Model file for the job. Use its own axes, mm. A direction names the side the tool comes from. Round coordinates to 2 decimals unless told otherwise and drop trailing zeros. Order: outer loops, then holes, each group sorted by start corner. A loop starts at its lowest first (then second) coordinate and runs counter-clockwise, first axis right, second up. Notation, with made-up numbers: (25.25, -4) - (73.25, -4) arc R10 cw to (73.25, 0) - close; hole circle Ø5 at (11.5, -38.5). An arc over 180 degrees is marked (long way). Answer as CSV lines item,"result". Start each with the question number.
1. Band-saw the part on C-C on y = -62. List the corners of the cut face in (x, z), then the cut area to 3 significant figures.
2. Pin check, flat tips, straight feed: pin 1 Ø1.5 at (x, z) = (2, 44) entering from +Y; pin 2 Ø3 at (y, z) = (-21.5, 20.5) entering from -X; pin 3 Ø1.5 at (x, y) = (1.5, -30) entering from +Z; pin 4 Ø1.5 at (x, z) = (3, -15.5) entering from +Y (3 decimals). Stop position of each tip, or through.
3. Band-saw the part on A-A on z = 45.5. List the corners of the cut face in (x, y), then the cut area to 3 significant figures.
4. Band-saw the part on D-D on y = -33. List the corners of the cut face in (x, z), then the cut area to 3 significant figures.
5. Wall check: line 1 along Y through (x, z) = (4, 0); line 2 along Z through (x, y) = (1, -30); line 3 along Y through (x, z) = (2.7, -17). Give the ranges that are in metal, low to high. Write a range as [from, to].
6. Band-saw the part on B-B on y = -17. List the corners of the cut face in (x, z), then the cut area to 3 significant figures.
7. 3-axis set-ups, long thin cutter, end or side, ignore diameter. For faces 1 (the face through (3, -34, 25.706)), 2 (the face through (5, -28.6, 7.8)): which of +Z, -Z, +X, -X, +Y, -Y reach the whole face in a straight line?
8. Pull direction Z, two halves, no side cores. Call faces 3 (the face through (2.54, -56.43, -11.4)), 4 (the face through (2, -32, -27)), 5 (the face through (3, -65, 19)): released by +Z, released by -Z, zero draft, split by the parting line, or undercut.
```python
from build123d import *

# Parameters (mm, degrees)
SKETCH_1_R           = 27
SKETCH_1_R_2         = 18.5
EXTRUDE_1_DEPTH      = 5
SKETCH_2_R           = 1.6
CUT_EXTRUDE_1_DEPTH  = 10
EXTRUDE_2_DEPTH      = 5
SKETCH_9_W           = 91
SKETCH_9_H           = 135
CUT_EXTRUDE_5_DEPTH  = 211.049994049
SKETCH_13_R          = 2.1
SKETCH_13_R_2        = 3.0525
CUT_EXTRUDE_6_DEPTH  = 92.356444764
SKETCH_14_R          = 1.6
CUT_EXTRUDE_7_DEPTH  = 92.356444764
SKETCH_15_W          = 24
SKETCH_15_H          = 9
CUT_EXTRUDE_8_DEPTH  = 10
FILLET_1_R           = 2
CUT_EXTRUDE_9_DEPTH  = 92.356444764
FILLET_2_R           = 1.3
CUT_EXTRUDE_10_DEPTH = 92.356444764
FILLET_3_R           = 1.3


with BuildPart() as part:
    # 草图1 → 凸台-拉伸1 (new body)
    with BuildSketch(Plane(origin=(0, 0, 0), x_dir=(0, 0, -1), z_dir=(1, 0, 0))):
        Circle(SKETCH_1_R)
        Circle(SKETCH_1_R_2, mode=Mode.SUBTRACT)
    extrude(amount=EXTRUDE_1_DEPTH)

    # 草图2 → 切除-拉伸1 (cut)
    with BuildSketch(Plane(origin=(5, 0, 0), x_dir=(0, 0, -1), z_dir=(1, 0, 0))):
        with Locations((23, 0)):
            Circle(SKETCH_2_R)
        with Locations((0, -23)):
            Circle(SKETCH_2_R)
        with Locations((0, 23)):
            Circle(SKETCH_2_R)
        with Locations((-23, 0)):
            Circle(SKETCH_2_R)
    extrude(amount=-CUT_EXTRUDE_1_DEPTH, mode=Mode.SUBTRACT)

    # 草图3 → 凸台-拉伸2 (add)
    with BuildSketch(Plane.ZY):
        with BuildLine():
            ThreePointArc((27, 0), (0, -27), (-27, 0))
            Line((-27, 0), (-27, -200))
            Line((-27, -200), (64, -200))
            Line((64, -200), (64, -60))
            Line((64, -60), (23.632414536, 13.057908838))
            ThreePointArc((23.632414536, 13.057908838), (26.144551942, 6.742581388), (27, 0))
        make_face()
    extrude(amount=-EXTRUDE_2_DEPTH)

    # 草图9 → 切除-拉伸5 (cut, through all)
    with BuildSketch(Plane(origin=(5, 0, 0), x_dir=(0, 0, -1), z_dir=(1, 0, 0))):
        with Locations((-18.5, -132.5)):
            Rectangle(SKETCH_9_W, SKETCH_9_H)
    extrude(amount=-CUT_EXTRUDE_5_DEPTH, mode=Mode.SUBTRACT)

    # 草图13 → 切除-拉伸6 (cut, through all)
    with BuildSketch(Plane(origin=(5, 0, 0), x_dir=(0, 0, -1), z_dir=(1, 0, 0))):
        with Locations((-17.5, -45)):
            Circle(SKETCH_13_R)
        with Locations((-17.5, -60)):
            Circle(SKETCH_13_R_2)
        with Locations((17.5, -60)):
            Circle(SKETCH_13_R_2)
        with Locations((17.5, -45)):
            Circle(SKETCH_13_R)
    extrude(amount=-CUT_EXTRUDE_6_DEPTH, mode=Mode.SUBTRACT)

    # 草图14 → 切除-拉伸7 (cut, through all)
    with BuildSketch(Plane.ZY):
        with Locations((39, -62)):
            Circle(SKETCH_14_R)
        with Locations((59, -62)):
            Circle(SKETCH_14_R)
    extrude(amount=-CUT_EXTRUDE_7_DEPTH, mode=Mode.SUBTRACT)

    # 草图15 → 切除-拉伸8 (cut)
    with BuildSketch(Plane.ZY):
        with Locations((0, -52.5)):
            Rectangle(SKETCH_15_W, SKETCH_15_H)
    extrude(amount=-CUT_EXTRUDE_8_DEPTH, mode=Mode.SUBTRACT)

    # 圆角1
    fillet_1_edges = [part.edges().sort_by_distance(p)[0] for p in [
        (2.5, -57, -12),
        (2.5, -48, -12),
        (2.5, -48, 12),
        (2.5, -57, 12),
    ]]
    fillet(fillet_1_edges, radius=FILLET_1_R)

    # 草图16 → 切除-拉伸9 (cut, through all)
    with BuildSketch(Plane(origin=(5, 0, 0), x_dir=(0, 0, -1), z_dir=(1, 0, 0))):
        with BuildLine():
            Line((-28.536090226, -9.256973298), (-52.705963097, -53))
            Line((-52.705963097, -53), (-25.705963097, -53))
            Line((-25.705963097, -53), (-25.705963097, -15.466203841))
            ThreePointArc((-25.705963097, -15.466203841), (-27.29814505, -12.442317985), (-28.536090226, -9.256973298))
        make_face()
    extrude(amount=-CUT_EXTRUDE_9_DEPTH, mode=Mode.SUBTRACT)

    # 圆角2
    fillet_2_edges = [part.edges().sort_by_distance(p)[0] for p in [
        (2.5, -9.256973298, 28.536090226),
        (2.5, -15.466203841, 25.705963097),
        (2.5, -53, 25.705963097),
        (2.5, -53, 52.705963097),
    ]]
    fillet(fillet_2_edges, radius=FILLET_2_R)

    # 草图17 → 切除-拉伸10 (cut, through all)
    with BuildSketch(Plane(origin=(5, 0, 0), x_dir=(0, 0, -1), z_dir=(1, 0, 0))):
        with BuildLine():
            ThreePointArc((-2.7, -29.878252961), (-8.364759165, -28.81025519), (-13.720671758, -26.678515073))
            Line((-13.720671758, -26.678515073), (-19.7, -37.5))
            Line((-19.7, -37.5), (-2.7, -37.5))
            Line((-2.7, -37.5), (-2.7, -29.878252961))
        make_face()
        with BuildLine():
            Line((19.7, -37.5), (13.720671758, -26.678515073))
            ThreePointArc((13.720671758, -26.678515073), (8.364759165, -28.81025519), (2.7, -29.878252961))
            Line((2.7, -29.878252961), (2.7, -37.5))
            Line((2.7, -37.5), (19.7, -37.5))
        make_face()
    extrude(amount=-CUT_EXTRUDE_10_DEPTH, mode=Mode.SUBTRACT)

    # 圆角3
    fillet_3_edges = [part.edges().sort_by_distance(p)[0] for p in [
        (2.5, -26.678515073, 13.720671758),
        (2.5, -29.878252961, 2.7),
        (2.5, -37.5, 2.7),
        (2.5, -37.5, 19.7),
        (2.5, -29.878252961, -2.7),
        (2.5, -26.678515073, -13.720671758),
        (2.5, -37.5, -19.7),
        (2.5, -37.5, -2.7),
    ]]
    fillet(fillet_3_edges, radius=FILLET_3_R)


solid = part.part
```
Reply:
1,outline,"(0, -27) - (5, -27) - (5, -19.81) - (0, -19.81) - close; (0, -15.19) - (5, -15.19) - (5, 15.19) - (0, 15.19) - close; (0, 19.81) - (5, 19.81) - (5, 37.4) - (0, 37.4) - close; (0, 40.6) - (5, 40.6) - (5, 57.4) - (0, 57.4) - close; (0, 60.6) - (5, 60.6) - (5, 64) - (0, 64) - close"
1,area,"377 mm2"
2,pin 1,"stops at y = -22.45"
2,pin 2,"stops at x = 0"
2,pin 3,"stops at z = 47.84"
2,pin 4,"stops at y = 22.615"
3,outline,"(0, -65) - (5, -65) - (5, -53) - (0, -53) - close; (0, -39.96) - (5, -39.96) - (5, -26.52) - (0, -26.52) - close"
3,area,"127 mm2"
4,outline,"(0, -27) - (5, -27) - (5, -17.21) - (0, -17.21) - close; (0, -2.7) - (5, -2.7) - (5, 2.7) - (0, 2.7) - close; (0, 17.21) - (5, 17.21) - (5, 25.71) - (0, 25.71) - close; (0, 41.66) - (5, 41.66) - (5, 49.08) - (0, 49.08) - close"
4,area,"156 mm2"
5,line 1,"y = [-65, -57], [-48, -24.6], [-21.4, -18.5], [18.5, 21.4], [24.6, 27]"
5,line 2,"z = [-27, -15.56], [-3.22, 3.22], [15.56, 25.71], [40, 47.42]"
5,line 3,"y = [-65, -63.01], [-56.99, -47.04], [-42.96, -37.5], [-32.61, -7.3], [7.3, 20.98]"
6,outline,"(0, -27) - (5, -27) - (5, -7.3) - (0, -7.3) - close; (0, 7.3) - (5, 7.3) - (5, 25.71) - (0, 25.71) - close; (0, 32.81) - (5, 32.81) - (5, 40.24) - (0, 40.24) - close"
6,area,"228 mm2"
7,face 1,"+X, -X"
7,face 2,"+Z, -Z, +X, +Y, -Y"
8,face 3,"undercut"
8,face 4,"released by -Z"
8,face 5,"zero draft"
